Check sheet for the modelled part. Datum: model origin and axes. Units: mm. A direction names the side the tool comes from. Round coordinates to 2 decimals unless told otherwise and drop trailing zeros. Write each loop counter-clockwise with the first axis right and the second up, starting at its lowest first coordinate (ties: lowest second). Pieces come first, ordered by that corner, then holes. Notation, with made-up numbers: (16, -22.5) -> (68, -22.5) arc R20 ccw to (68, -2.5) -> close; hole circle Ø6 at (-16.75, -10.5). An arc over 180 degrees is marked (long way). Write item = value, one per line.
from build123d import *

# Parameters (mm, degrees)
F3_DEPTH = 70
F4_R     = 30
F5_DEPTH = 112
F6_R     = 15
F7_DEPTH = 163
F9_DEPTH = 150


with BuildPart() as f2:
    # F1 (on Front) → F2 (revolve)
    with BuildSketch(Plane.XZ):
        Polygon((-60, -120), (-60, -250), (0, -250), (0, 0), (-70, 0), (-70, -120), align=None)
    revolve(axis=Axis((0, 0, -125), (0, 0, -1)))

    # F0 (on Front) → F3 (join, symmetric)
    with BuildSketch(Plane.XZ):
        with BuildLine():
            ThreePointArc((113.275358, 0), (147.343032, 146.027594), (242.512075, 261.904762))
            ThreePointArc((242.512075, 261.904762), (192.752359, 769.029387), (-240, 500))
            Line((-240, 500), (-125, 500))
            ThreePointArc((-125, 500), (-95.197164, 581.009259), (-20, 623.389627))
            Line((-20, 623.389627), (-20, 624.947867))
            Line((-20, 624.947867), (20, 624.947867))
            Line((20, 624.947867), (20, 623.389627))
            ThreePointArc((20, 623.389627), (97.236318, 578.549974), (124.836727, 493.613169))
            Line((124.836727, 493.613169), (0, 278.411619))
            Line((0, 278.411619), (-31.669397, 232.573897))
            ThreePointArc((-31.669397, 232.573897), (-58.197727, 223.86417), (-66.061109, 197.072774))
            Line((-66.061109, 197.072774), (-66.061109, 164.52672))
            ThreePointArc((-66.061109, 164.52672), (-98.826102, 85.146444), (-110, 0))
            Line((-110, 0), (113.275358, 0))
        make_face()
        with BuildLine():
            Line((-125, 500), (-240, 500))
            Line((-240, 500), (-240, 350))
            ThreePointArc((-240, 350), (-219.930134, 325.490945), (-191.944498, 340.333365))
            Line((-191.944498, 340.333365), (-125, 500))
        make_face()
    extrude(amount=F3_DEPTH, both=True)

    # F4 (on Front) → F5 (cut, symmetric)
    with BuildSketch(Plane.XZ):
        with Locations((0, -190)):
            Circle(F4_R)
    extrude(amount=F5_DEPTH, both=True, mode=Mode.SUBTRACT)

    # F6 (on face) → F7 (cut, symmetric)
    with BuildSketch(Plane.XZ.offset(70)):
        with Locations((-43.483209, 207.776994)):
            Circle(F6_R)
    extrude(amount=F7_DEPTH, both=True, mode=Mode.SUBTRACT)

    # F8 (on face) → F9 (cut)
    with BuildSketch(Plane.XZ.offset(70)):
        with BuildLine():
            ThreePointArc((207.243012, 533.562227), (251.876022, 519.636331), (279.226912, 557.556839))
            ThreePointArc((279.226912, 557.556839), (68.171297, 754.813507), (-170.094242, 591.460519))
            ThreePointArc((-170.094242, 591.460519), (-171.994625, 567.583929), (-148.132823, 565.506094))
            ThreePointArc((-148.132823, 565.506094), (41.282548, 680.00219), (207.243012, 533.562227))
        make_face()
    extrude(amount=-F9_DEPTH, mode=Mode.SUBTRACT)


solid = f2.part
(1) Release check for a two-part mould opening along Z. For faces 4 (the flat face through (63.292, -0.98, 387.519)), 5 (the cylindrical face through (200.34, -0.98, 765.15)), 6 (the flat face through (-80, -1, 0)) record: pulls with the +Z half, pulls with the -Z half, needs draft (parallel to the pull), parting line crosses it, or undercut.
Worked answers:
face_4 = undercut
face_5 = parting line crosses it
face_6 = pulls with the -Z half
(2) Sectioned sample at C-C on z = -37. Enter the section's corners in (x, y).
Worked answers:
outline = circle Ø140 at (0, 0)
(3) Sectioned sample at B-B on y = -14. Count the separate pieces of the cut face and the enclosed holes in it, then the cut area to 3 significant figures.
Worked answers:
separate_pieces = 1
enclosed_holes = 3
area = 243,000 mm²
(4) Material ranges on L1, parallel to X at y = 16, z = 603; L2, parallel to X at y = 3, z = -190; L3, parallel to Z at x = -67.5, y = 32, recorded low to high. Write a range as [from, to].
Worked answers:
L1 = [-221.76, -166.27], [-127.22, -70.82], [70.82, 176.3], [267.89, 341.76]
L2 = [-59.92, -30], [30, 59.92]
L3 = [0, 162], [605.21, 656.53], [722.83, 771.56]
(5) Access from +Z, -Z, +X, -X, +Y, -Y to the whole of each face (thin tool, end or side, straight path). Record for faces 1 (the flat face through (-66.061, -1, 181)), 2 (the flat face through (-52, 31, -120)), 3 (the cylindrical face through (-95.99, -0.98, 580.07)).
Worked answers:
face_1 = -X, +Y, -Y
face_2 = -Z
face_3 = +Y, -Y
(6) Sectioned sample at D-D on z = -190. Enter the section's corners in (x, y), then the cut area to 3 significant figures.
Worked answers:
outline = (-30, -51.96) -> (-30, 51.96) arc R60 ccw to start; (30, -51.96) arc R60 ccw to (30, 51.96) -> close
area = 4,420 mm²
(7) Go/stop test with flat-tipped pins: P1, Ø16.5, axis at y = -33, z = 177, coming from the -X side; P2, Ø1.5, axis at y = 3.5, z = 535, coming from the -X side; P3, Ø8, axis at x = 9, y = 39, coming from the +Z side. Record where each tip stops, or that it passes through.
Worked answers:
P1 = -66.06
P2 = -238.04
P3 = 796.3
(8) Sectioned sample at A-A on x = -80.5. Enter the section's corners in (y, z).
Worked answers:
outline = (-70, 0) -> (70, 0) -> (70, 136.38) -> (-70, 136.38) -> close; (-70, 595.63) -> (70, 595.63) -> (70, 648.46) -> (-70, 648.46) -> close; (-70, 714.47) -> (70, 714.47) -> (70, 765.07) -> (-70, 765.07) -> close
